Autodesk Fusion 360 part; units mm, degrees
sketch "Sketch1" plane through (0, 0, 0) normal (0, 0, 1) x (1, 0, 0)
  line L0 (9.2315, 7.937) -> (25.5856, 13.6416)
  line L1 (25.5856, 13.6416) -> (38.703, 2.3308)
  line L2 (38.703, 2.3308) -> (35.4663, -14.6846)
  line L3 (35.4663, -14.6846) -> (19.1122, -20.3892)
  line L4 (19.1122, -20.3892) -> (5.9948, -9.0784)
  line L5 (5.9948, -9.0784) -> (9.2315, 7.937)
  circle A0 centre (22.3489, -3.3738) radius 1.75
  dimension "d1" = 120
  dimension "d2" = 120
  dimension "d3" = 120
  dimension "d4" = 120
  dimension "d5" = 120
  dimension "d6" = 30
  dimension "d7" = 30
  dimension "d8" = 30
  dimension "d9" = 3.5
extrude "Extrude1" add sketch "Sketch1" along normal blind 5
fillet "Fillet1" radius 5 1 edges at (20.7173, -2.741, 5)
For this review, take the finished solid that the model builds, in its own axes (mm). Give positions to 0.01 mm unless a question says otherwise; leave off trailing zeros. Loops run counter-clockwise (first coordinate to the right, second up) from the corner with the lowest first, then second, coordinate; pieces in that order, holes last. Notation, with made-up numbers: M -33.5,-9 L -2.5,-9 A19 cw -2.5,19 Z; hole C 12,44 d10. An arc over 180 degrees is marked long. Answer as a JSON object with one key per item and string values. Group by question number.
Q1. Insertion check: P1, Ø1, axis at y = -0.5, z = 3.5, coming from the -X side; P2, Ø3, axis at x = 32, z = 1, coming from the +Y side; P3, Ø1, axis at x = 10, z = 4, coming from the -Y side; P4, Ø2, axis at x = 22.35, y = -3.37, coming from the +Z side. Each pin has a flat end and moves straight along its axis. Give the tip position at first contact, or say it passes through.
Q2. Add section C-C on x = 12. Give the boundary of the cut face in (y, z), and give its area (3 significant figures).
Q3. For probe 1 along Y at (x, z) = (22, 2.45); probe 2 along Y at (x, z) = (24, 1.4); probe 3 along X at (y, z) = (-9, 1.6), list the stretches that pass through material, from the lowest coordinate up. Write a range as [from, to].
Q4. Add section A-A on z = 2.5. Give the boundary of the cut face in (x, y).
Q5. Add section D-D on x = 32. Give the boundary of the cut face in (y, z).
Q6. Add section B-B on z = 4.55. Give the boundary of the cut face in (x, y), and give its area (3 significant figures).
Checked values:
{
 "1": {"P1": "x = 7.53", "P2": "y = 9.4", "P3": "y = -12.96", "P4": "through"},
 "2": {"outline": "M -14.26,0 L 8.9,0 L 8.9,5 L -14.26,5 Z", "area": "116 mm²"},
 "3": {"probe 1": "[-19.38, -5.74], [-1.01, 12.39]", "probe 2": "[-18.68, -4.41], [-2.34, 13.09]", "probe 3": "[6.01, 36.55]"},
 "4": {"outline": "M 5.99,-9.08 L 19.11,-20.39 L 35.47,-14.68 L 38.7,2.33 L 25.59,13.64 L 9.23,7.94 Z; hole C 22.35,-3.37 d4.84"},
 "5": {"outline": "M -15.89,0 L 8.11,0 L 8.11,5 L -15.89,5 Z"},
 "6": {"outline": "M 5.99,-9.08 L 19.11,-20.39 L 35.47,-14.68 L 38.7,2.33 L 25.59,13.64 L 9.23,7.94 Z; hole C 22.35,-3.37 d9.35", "area": "711 mm²"}
}
